```python
from build123d import *

# Parameters (mm, degrees)
F1_DEPTH = 3
F2_SIZE  = 30


with BuildPart() as f1:
    # F0 (on Front) → F1 (new body, symmetric)
    with BuildSketch(Plane.XZ):
        Polygon((0, -50), (0, 50), (-118.5, 50), (-118.5, 0), (-96.60254, 0), (-10, -50), align=None)
    extrude(amount=F1_DEPTH, both=True)

    # F2
    f2_edges = [f1.edges().sort_by_distance(p)[0] for p in [
        (-118.5, 0, 50),
    ]]
    chamfer(f2_edges, length=F2_SIZE)


solid = f1.part
```
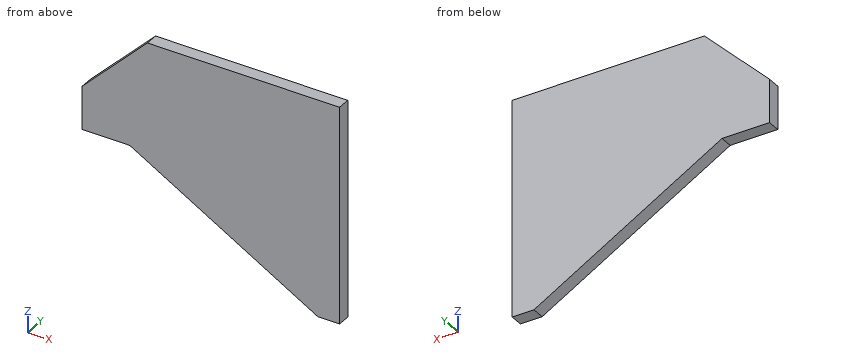
Part model, mm, in its own coordinate system. Give positions to 0.01 mm unless a question says otherwise; leave off trailing zeros. Write each loop counter-clockwise with the first axis right and the second up, starting at its lowest first coordinate (ties: lowest second). Pieces come first, ordered by that corner, then holes. Notation, with made-up numbers: (52, 47.5) -> (93, 47.5) arc R22 cw to (93, 83.5) -> close; hole circle Ø1 at (43, 51). An arc over 180 degrees is marked (long way). Put each result on its own line as item: value. Start each with the question number.
Item 1: Cut at A-A (y = -0.25). List the corners of the cut face in (x, z).
Item 2: Cut at B-B (z = 37). List the corners of the cut face in (x, y), then the cut area to 3 significant figures.
Item 3: Wall check: L1, parallel to X at y = 1, z = -44; L2, parallel to Z at x = -48, y = 2; L3, parallel to X at y = 1.25, z = -2.5. Give the ranges that are in metal, low to high. Write a range as [from, to].
Item 4: Pin check, flat tip, straight feed: pin 1 Ø1.8 at (x, y) = (-102, 1) entering from -Z. Stop position of the tip, or through.
Item 5: Cut at C-C (x = -109.5). List the corners of the cut face in (y, z), then the cut area to 3 significant figures.
Answer list:
1. outline: (-118.5, 0) -> (-96.6, 0) -> (-10, -50) -> (0, -50) -> (0, 50) -> (-88.5, 50) -> (-118.5, 20) -> close
2. outline: (-101.5, -3) -> (0, -3) -> (0, 3) -> (-101.5, 3) -> close
2. area: 609 mm2
3. L1: x = [-20.39, 0]
3. L2: z = [-28.06, 50]
3. L3: x = [-92.27, 0]
4. pin 1: stops at z = 0
5. outline: (-3, 0) -> (3, 0) -> (3, 29) -> (-3, 29) -> close
5. area: 174 mm2
